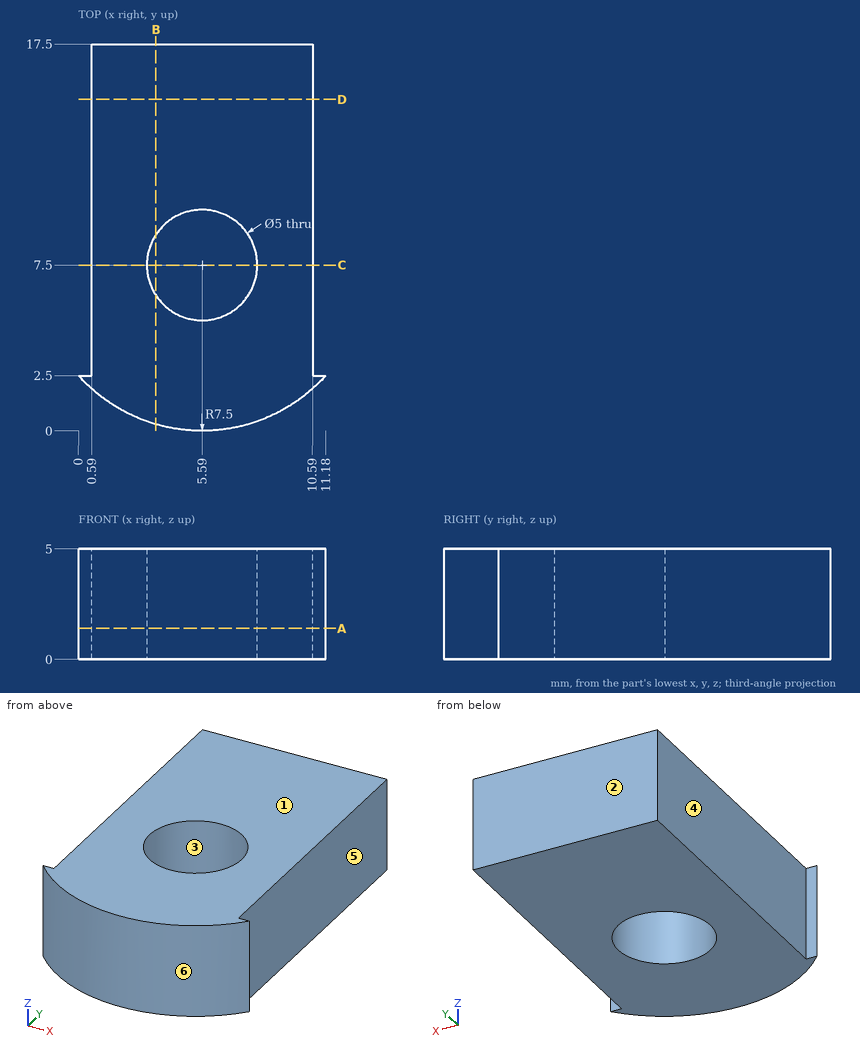
Input: dimensioned drawing with shaded views. Units: mm. Origin: part minimum x, y, z. A direction names the side the tool comes from. Give positions to 0.01 mm unless a question says otherwise; leave off trailing zeros. Write each loop counter-clockwise with the first axis right and the second up, starting at its lowest first coordinate (ties: lowest second). Pieces come first, ordered by that corner, then holes.
1. Pull-direction query (Y, two-part tool) for the marked faces 1, 2 and 3; classes: +Y half, -Y half, draft (parallel to the pull), parting line (faces both ways), or undercut.
2. Section query C-C (y = 7.5). Return the cut outline in (x, z), then the cut area to 3 significant figures.
3. Section query D-D (y = 15). Return the cut outline in (x, z).
4. Access query for the marked faces 4, 5 and 6. Directions: +Z, -Z, +X, -X, +Y, -Y. A direction counts if a zero-diameter tool reaches every point of the face in a straight line with its end or side. Return the directions, or none.
5. Material intervals for line 1 along Y through (x, z) = (6.75, 2.8) (1 decimal); line 2 along Y through (x, z) = (5.5, 3.9); line 3 along X through (y, z) = (3.75, 1.95), sorted ascending.
6. First-contact query: pin 1 (2.5 mm diameter, centred on y = 13.5, z = 3.5, fed in from +X); pin 2 (0.5 mm diameter, centred on x = 11, z = 2.5, fed in from +Y); pin 3 (4 mm diameter, centred on x = 5.59, y = 7.5, fed in from -Z); pin 4 (1.5 mm diameter, centred on y = 8.5, z = 3, fed in from -X). Flat tips, straight axial feed; report the tip coordinate or a pass-through.
7. Section query B-B (x = 3.5). Return the cut outline in (y, z), then the cut area to 3 significant figures.
8. Section query A-A (z = 1.4). Return the cut outline in (x, y), then the cut area to 3 significant figures.
Output values:
1. face 1: draft
1. face 2: +Y half
1. face 3: undercut
2. outline: (0.59, 0) - (3.09, 0) - (3.09, 5) - (0.59, 5) - close; (8.09, 0) - (10.59, 0) - (10.59, 5) - (8.09, 5) - close
2. area: 25.0 mm2
3. outline: (0.59, 0) - (10.59, 0) - (10.59, 5) - (0.59, 5) - close
4. face 4: +Z, -Z, -X, +Y
4. face 5: +Z, -Z, +X, +Y
4. face 6: +Z, -Z, -Y
5. line 1: y = 0.1 to 5.3, 9.7 to 17.5
5. line 2: y = 0 to 5, 10 to 17.5
5. line 3: x = 0.59 to 10.59
6. pin 1: stops at x = 10.59
6. pin 2: stops at y = 2.5
6. pin 3: passes through
6. pin 4: stops at x = 0.59
7. outline: (0.3, 0) - (6.13, 0) - (6.13, 5) - (0.3, 5) - close; (8.87, 0) - (17.5, 0) - (17.5, 5) - (8.87, 5) - close
7. area: 72.3 mm2
8. outline: (0, 2.5) arc R7.5 ccw to (11.18, 2.5) - (10.59, 2.5) - (10.59, 17.5) - (0.59, 17.5) - (0.59, 2.5) - close; hole circle Ø5 at (5.59, 7.5)
8. area: 150 mm2
